```python
from build123d import *

# Parameters (mm, degrees)
CROQUIS1_W              = 330
CROQUIS1_H              = 303.31
SALIENTE_EXTRUIR2_DEPTH = 6.35
CROQUIS4_R              = 3.96875
CORTAR_EXTRUIR1_DEPTH   = 10


with BuildPart() as part:
    # Croquis1 → Saliente-Extruir2 (new body)
    with BuildSketch(Plane(origin=(0, 0, 0), x_dir=(1, 0, 0), z_dir=(0, 1, 0))):
        Rectangle(CROQUIS1_W, CROQUIS1_H)
    extrude(amount=SALIENTE_EXTRUIR2_DEPTH)

    # Croquis4 → Cortar-Extruir1 (cut)
    with BuildSketch(Plane(origin=(0, 6.35, 0), x_dir=(1, 0, 0), z_dir=(0, 1, 0))):
        with Locations(Location((122.58, -128.507, 0), (0, 0, 270))):
            Circle(CROQUIS4_R)
        with Locations(Location((122.58, -115.807, 0), (0, 0, 270))):
            Circle(CROQUIS4_R)
        with Locations(Location((122.58, -141.207, 0), (0, 0, 270))):
            Circle(CROQUIS4_R)
        with Locations(Location((71.78, -141.207, 0), (0, 0, 270))):
            Circle(CROQUIS4_R)
        with Locations(Location((71.78, -128.507, 0), (0, 0, 270))):
            Circle(CROQUIS4_R)
        with Locations(Location((71.78, -115.807, 0), (0, 0, 270))):
            Circle(CROQUIS4_R)
        with Locations(Location((95.15, -36.499, 0), (0, 0, 270))):
            Circle(CROQUIS4_R)
        with Locations(Location((95.15, -23.799, 0), (0, 0, 270))):
            Circle(CROQUIS4_R)
        with Locations(Location((95.15, -49.199, 0), (0, 0, 270))):
            Circle(CROQUIS4_R)
        with Locations(Location((145.95, -49.199, 0), (0, 0, 270))):
            Circle(CROQUIS4_R)
        with Locations(Location((145.95, -36.499, 0), (0, 0, 270))):
            Circle(CROQUIS4_R)
        with Locations(Location((145.95, -23.799, 0), (0, 0, 270))):
            Circle(CROQUIS4_R)
        with Locations(Location((145.95, 49.199, 0), (0, 0, 270))):
            Circle(CROQUIS4_R)
        with Locations(Location((95.15, 49.199, 0), (0, 0, 270))):
            Circle(CROQUIS4_R)
        with Locations(Location((145.95, 36.499, 0), (0, 0, 270))):
            Circle(CROQUIS4_R)
        with Locations(Location((95.15, 36.499, 0), (0, 0, 270))):
            Circle(CROQUIS4_R)
        with Locations(Location((145.95, 23.799, 0), (0, 0, 270))):
            Circle(CROQUIS4_R)
        with Locations(Location((95.15, 23.799, 0), (0, 0, 270))):
            Circle(CROQUIS4_R)
        with Locations(Location((-95.15, -49.199, 0), (0, 0, 270))):
            Circle(CROQUIS4_R)
        with Locations(Location((-145.95, -49.199, 0), (0, 0, 270))):
            Circle(CROQUIS4_R)
        with Locations(Location((-145.95, -36.499, 0), (0, 0, 270))):
            Circle(CROQUIS4_R)
        with Locations(Location((-95.15, -36.499, 0), (0, 0, 270))):
            Circle(CROQUIS4_R)
        with Locations(Location((-95.15, -23.799, 0), (0, 0, 270))):
            Circle(CROQUIS4_R)
        with Locations(Location((-145.95, -23.799, 0), (0, 0, 270))):
            Circle(CROQUIS4_R)
        with Locations(Location((-145.95, 49.199, 0), (0, 0, 270))):
            Circle(CROQUIS4_R)
        with Locations(Location((-145.95, 36.499, 0), (0, 0, 270))):
            Circle(CROQUIS4_R)
        with Locations(Location((-145.95, 23.799, 0), (0, 0, 270))):
            Circle(CROQUIS4_R)
        with Locations(Location((-95.15, 23.799, 0), (0, 0, 270))):
            Circle(CROQUIS4_R)
        with Locations(Location((-95.15, 36.499, 0), (0, 0, 270))):
            Circle(CROQUIS4_R)
        with Locations(Location((-95.15, 49.199, 0), (0, 0, 270))):
            Circle(CROQUIS4_R)
        with Locations(Location((-122.58, 115.807, 0), (0, 0, 270))):
            Circle(CROQUIS4_R)
        with Locations(Location((-122.58, 128.507, 0), (0, 0, 270))):
            Circle(CROQUIS4_R)
        with Locations(Location((-122.58, 141.207, 0), (0, 0, 270))):
            Circle(CROQUIS4_R)
        with Locations(Location((-71.78, 115.807, 0), (0, 0, 270))):
            Circle(CROQUIS4_R)
        with Locations(Location((-71.78, 128.507, 0), (0, 0, 270))):
            Circle(CROQUIS4_R)
        with Locations(Location((-71.78, 141.207, 0), (0, 0, 270))):
            Circle(CROQUIS4_R)
    extrude(amount=-CORTAR_EXTRUIR1_DEPTH, mode=Mode.SUBTRACT)


solid = part.part
```
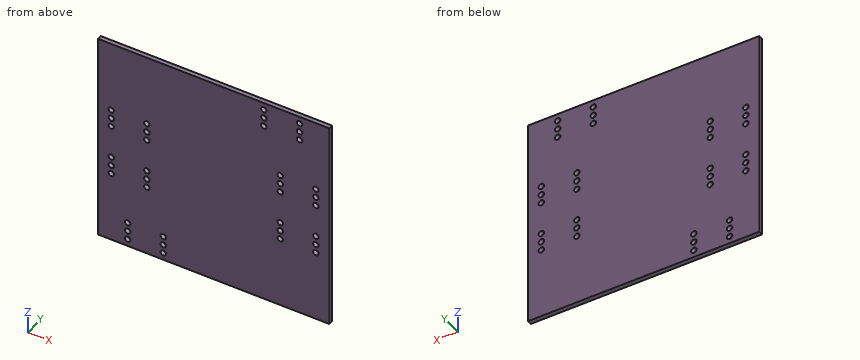
Input: part model. Units: mm. Frame: model coordinates. Coordinates: 2 decimals unless noted, no trailing zeros. Loops run counter-clockwise (first coordinate to the right, second up) from the corner with the lowest first, then second, coordinate; pieces in that order, holes last.
Q1. Section C-C, the plane y = 1.75. Give the number of separate pieces and of enclosed holes in the cut face, and give its area (3 significant figures).
Results are:
separate pieces: 1
enclosed holes: 36
area: 98,300 mm2
Q2. Section B-B, the plane x = -71.78. Return the cut outline in (y, z) (3 decimals).
Results are:
outline: (0, -151.655) - (6.35, -151.655) - (6.35, -145.176) - (0, -145.176) - close; (0, -137.238) - (6.35, -137.238) - (6.35, -132.476) - (0, -132.476) - close; (0, -124.538) - (6.35, -124.538) - (6.35, -119.776) - (0, -119.776) - close; (0, -111.838) - (6.35, -111.838) - (6.35, 151.655) - (0, 151.655) - close
Q3. Section A-A, the plane x = -145.95. Return the cut outline in (y, z) (3 decimals).
Results are:
outline: (0, -151.655) - (6.35, -151.655) - (6.35, -53.168) - (0, -53.168) - close; (0, -45.23) - (6.35, -45.23) - (6.35, -40.468) - (0, -40.468) - close; (0, -32.53) - (6.35, -32.53) - (6.35, -27.768) - (0, -27.768) - close; (0, -19.83) - (6.35, -19.83) - (6.35, 19.83) - (0, 19.83) - close; (0, 27.768) - (6.35, 27.768) - (6.35, 32.53) - (0, 32.53) - close; (0, 40.468) - (6.35, 40.468) - (6.35, 45.23) - (0, 45.23) - close; (0, 53.168) - (6.35, 53.168) - (6.35, 151.655) - (0, 151.655) - close
Q4. Line query: line 1 along X through (y, z) = (3, 129); line 2 along X through (y, z) = (3.5, -129.5); line 3 along X through (y, z) = (1.5, 25.5). Output: solid intervals per line, ascending.
Results are:
line 1: x = -165 to 67.84, 75.72 to 118.64, 126.52 to 165
line 2: x = -165 to -126.42, -118.74 to -75.62, -67.94 to 165
line 3: x = -165 to -149.54, -142.36 to -98.74, -91.56 to 91.56, 98.74 to 142.36, 149.54 to 165
